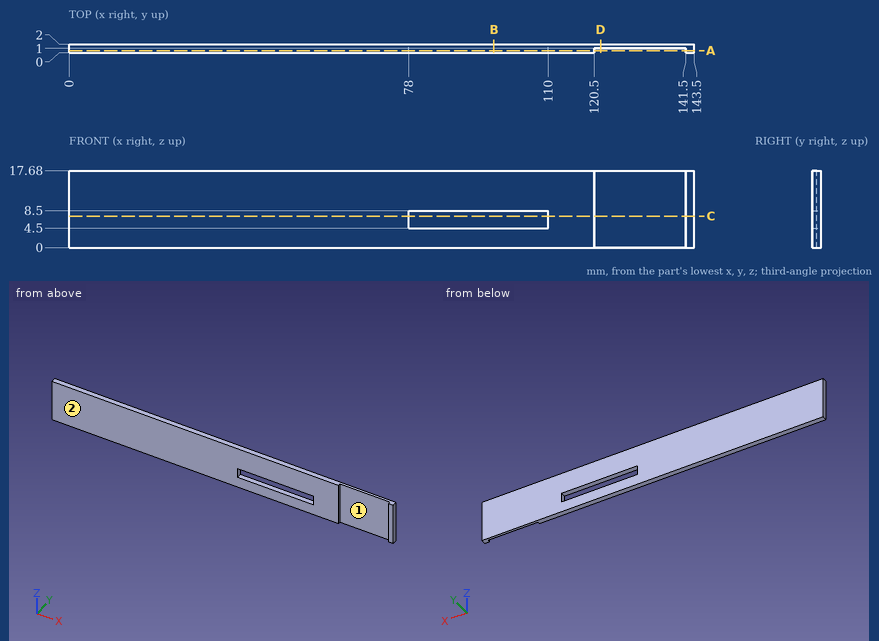
Geometry: see drawing. Coordinates: mm, zero at the bounding-box minimum. A direction names the side the tool comes from. Give positions to 0.01 mm unless a question says otherwise; leave off trailing zeros. Loops run counter-clockwise (first coordinate to the right, second up) from the corner with the lowest first, then second, coordinate; pieces in that order, holes last. Notation, with made-up numbers: (-14, -30.75) - (5, -30.75) arc R28 cw to (5, 4.25) - close; hole circle Ø11 at (-1, 22). An arc over 180 degrees is marked (long way). Use CSV: the item, a comma, the result in double quotes.
1) Set-up query: the marked faces 1 and 2. Return all of +Z, -Z, +X, -X, +Y, -Y with unobstructed straight access to the full face (end or side cutting, diameter ignored); none if empty.
Worked out:
face 1,"+Z, -Z, -Y"
face 2,"+Z, -Z, +X, -X, -Y"
2) Cut plane C-C (z = 7.25). Output: boundary loops of the cut face in (x, y).
Worked out:
outline,"(0, 0) - (78, 0) - (78, 2) - (0, 2) - close; (110, 0) - (120.5, 0) - (120.5, 1) - (141.5, 1) - (141.5, 0) - (143.5, 0) - (143.5, 2) - (110, 2) - close"
3) Cut plane D-D (x = 122). Output: boundary loops of the cut face in (y, z), and give its area (3 significant figures).
Worked out:
outline,"(1, 0) - (2, 0) - (2, 17.68) - (1, 17.68) - close"
area,"17.7 mm^2"
4) Line query: line 1 (X direction, y = 0.5, z = 6.5); line 2 (Z direction, x = 90, y = 1.15); line 3 (X direction, y = 0.5, z = 10.5). Output: solid intervals per line, ascending.
Worked out:
line 1,"x = 0 to 78, 110 to 120.5, 141.5 to 143.5"
line 2,"z = 0 to 4.5, 8.5 to 17.68"
line 3,"x = 0 to 120.5, 141.5 to 143.5"
5) Cut plane A-A (y = 0.5). Output: boundary loops of the cut face in (x, z).
Worked out:
outline,"(0, 0) - (120.5, 0) - (120.5, 17.68) - (0, 17.68) - close; (141.5, 0) - (143.5, 0) - (143.5, 17.68) - (141.5, 17.68) - close; hole (78, 4.5) - (110, 4.5) - (110, 8.5) - (78, 8.5) - close"
6) Pin query (flat end, axial travel): P1, Ø9, axis at x = 130.5, z = 9, coming from the -Y side. Return the tip coordinate at first contact, or that it passes through.
Worked out:
P1,"stops at y = 1"
7) Cut plane B-B (x = 97.5). Output: boundary loops of the cut face in (y, z).
Worked out:
outline,"(0, 0) - (2, 0) - (2, 4.5) - (0, 4.5) - close; (0, 8.5) - (2, 8.5) - (2, 17.68) - (0, 17.68) - close"
